The model under review builds one solid part; all positions refer to its coordinate system, in mm. Coordinates: 2 decimals unless noted, no trailing zeros. Use one line per item in the form item = value.
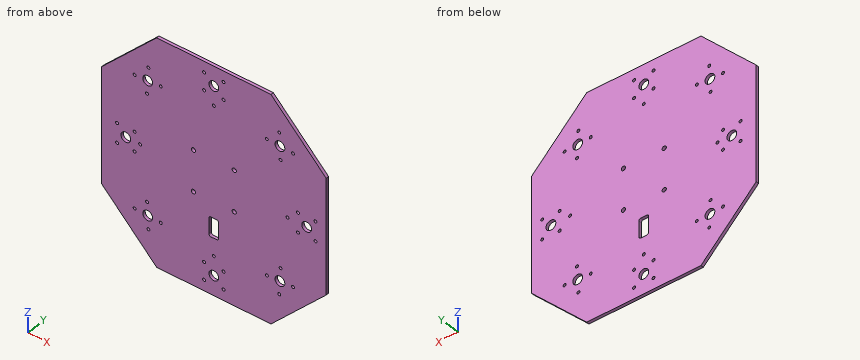
from build123d import *

# Parameters (mm, degrees)
SKETCH1_W                        = 230
SKETCH1_H                        = 230
BOSS_EXTRUDE1_DEPTH              = 3
CHAMFER2_START                   = -1
CHAMFER2_OUTLINE_W               = 82
CHAMFER2_OUTLINE_H               = 3
CHAMFER2_DEPTH                   = 40.999969952
CHAMFER3_START                   = -164
CHAMFER3_OUTLINE_W               = 83
CHAMFER3_OUTLINE_H               = 3
CHAMFER3_DEPTH                   = 41.365410279
CHAMFER4_START                   = 285.269149394
CHAMFER4_OUTLINE_W               = 82
CHAMFER4_OUTLINE_H               = 3
CHAMFER4_DEPTH                   = 40.730850606
CHAMFER5_START                   = 122.634589721
CHAMFER5_OUTLINE_W               = 83
CHAMFER5_OUTLINE_H               = 3
CHAMFER5_DEPTH                   = 41.365410279
F_11_64_0_17188_DIAMETER_HOLE1_D = 4.365752
CUT_EXTRUDE3_DEPTH               = 326.28295375
FILLET9_R                        = 2
FILLET10_R                       = 2
FILLET11_R                       = 2
FILLET12_R                       = 2
F_10_0MM_DOWEL_HOLE1_D           = 10
F_3_0MM_DOWEL_HOLE1_D            = 3
F_3_0MM_DOWEL_HOLE2_D            = 3


with BuildPart() as part:
    # Sketch1 → Boss-Extrude1 (new body)
    with BuildSketch(Plane(origin=(0, 0, 0), x_dir=(1, 0, 0), z_dir=(0, 1, 0))):
        with Locations((115, 115)):
            Rectangle(SKETCH1_W, SKETCH1_H)
    extrude(amount=BOSS_EXTRUDE1_DEPTH)

    # Chamfer2: read off the stored shape, not the designer's step
    # Chamfer2 outline → Chamfer2 (cut)
    with BuildSketch(Plane(origin=(0, 0, 0), x_dir=(0.7071067811865474, 0, 0.7071067811865477), z_dir=(0.7071067811865476, 0, -0.7071067811865476)).offset(CHAMFER2_START)):
        with Locations((0, -1.5)):
            Rectangle(CHAMFER2_OUTLINE_W, CHAMFER2_OUTLINE_H)
    extrude(amount=CHAMFER2_DEPTH, mode=Mode.SUBTRACT)

    # Chamfer3: read off the stored shape, not the designer's step
    # Chamfer3 outline → Chamfer3 (cut)
    with BuildSketch(Plane(origin=(0, 0, 0), x_dir=(0.7071067811865474, 0, -0.7071067811865477), z_dir=(0.7071067811865476, 0, 0.7071067811865476)).offset(CHAMFER3_START)):
        with Locations((162.5, 1.5)):
            Rectangle(CHAMFER3_OUTLINE_W, CHAMFER3_OUTLINE_H)
    extrude(amount=CHAMFER3_DEPTH, mode=Mode.SUBTRACT)

    # Chamfer4: read off the stored shape, not the designer's step
    # Chamfer4 outline → Chamfer4 (cut)
    with BuildSketch(Plane(origin=(0, 0, 0), x_dir=(0.7071067811865474, 0, 0.7071067811865477), z_dir=(0.7071067811865476, 0, -0.7071067811865476)).offset(CHAMFER4_START)):
        with Locations((0, -1.5)):
            Rectangle(CHAMFER4_OUTLINE_W, CHAMFER4_OUTLINE_H)
    extrude(amount=CHAMFER4_DEPTH, mode=Mode.SUBTRACT)

    # Chamfer5: read off the stored shape, not the designer's step
    # Chamfer5 outline → Chamfer5 (cut)
    with BuildSketch(Plane(origin=(0, 0, 0), x_dir=(0.7071067811865471, 0, -0.707106781186548), z_dir=(0.707106781186548, 0, 0.707106781186547)).offset(CHAMFER5_START)):
        with Locations((162.5, 1.5)):
            Rectangle(CHAMFER5_OUTLINE_W, CHAMFER5_OUTLINE_H)
    extrude(amount=CHAMFER5_DEPTH, mode=Mode.SUBTRACT)

    # 11/64 (0.17188) Diameter Hole1 (through all)
    with Locations(Plane(origin=(0, 3, 0), x_dir=(1, 0, 0), z_dir=(0, 1, 0))):
        with Locations((94.140349955, 135.859650045), (135.859650045, 135.859650045), (135.859650045, 94.140349955), (94.140349955, 94.140349955)):
            Hole(F_11_64_0_17188_DIAMETER_HOLE1_D / 2)

    # Sketch11 → Cut-Extrude3 (cut, through all)
    with BuildSketch(Plane(origin=(0, 3, 0), x_dir=(1, 0, 0), z_dir=(0, 1, 0))):
        Polygon((115, 152.5), (120, 152.5), (120, 172.5), (110, 172.5), (110, 152.5), align=None)
    extrude(amount=-CUT_EXTRUDE3_DEPTH, mode=Mode.SUBTRACT)

    # Fillet9
    fillet9_edges = [part.edges().sort_by_distance(p)[0] for p in [
        (120, 1.5, -172.5),
    ]]
    fillet(fillet9_edges, radius=FILLET9_R)

    # Fillet10
    fillet10_edges = [part.edges().sort_by_distance(p)[0] for p in [
        (110, 1.5, -172.5),
    ]]
    fillet(fillet10_edges, radius=FILLET10_R)

    # Fillet11
    fillet11_edges = [part.edges().sort_by_distance(p)[0] for p in [
        (120, 1.5, -152.5),
    ]]
    fillet(fillet11_edges, radius=FILLET11_R)

    # Fillet12
    fillet12_edges = [part.edges().sort_by_distance(p)[0] for p in [
        (110, 1.5, -152.5),
    ]]
    fillet(fillet12_edges, radius=FILLET12_R)

    # Ø10.0mm Dowel Hole1 (through all)
    with Locations(Plane(origin=(0, 3, 0), x_dir=(1, 0, 0), z_dir=(0, 1, 0))):
        with Locations((210, 115), (182.623866908, 182.623866908), (182.623866908, 47.376133092), (115, 20), (47.376133092, 47.376133092), (25, 115), (47.376133092, 182.623866908), (115, 210)):
            Hole(F_10_0MM_DOWEL_HOLE1_D / 2)

    # Ø3.0mm Dowel Hole1 (through all)
    with Locations(Plane(origin=(0, 0, 0), x_dir=(-1, 0, 0), z_dir=(0, -1, 0))):
        with Locations((-201.05, 124.95), (-201.05, 105.05), (-218.95, 124.95), (-218.95, 105.05), (-183.330973689, 60.740451256), (-169.259548744, 46.669026311), (-181.916760127, 34.011814928), (-195.988185072, 48.083239873), (-183.330973689, 169.259548744), (-169.259548744, 183.330973689), (-181.916760127, 195.988185072), (-195.988185072, 181.916760127), (-124.95, 201.05), (-124.95, 218.95), (-105.05, 218.95), (-105.05, 201.05), (-60.740451256, 183.330973689), (-34.011814928, 181.916760127), (-46.669026311, 169.259548744), (-48.083239873, 195.988185072), (-16.05, 124.95), (-33.95, 105.05), (-33.95, 124.95), (-16.05, 105.05), (-60.740451256, 46.669026311), (-48.083239873, 34.011814928), (-46.669026311, 60.740451256), (-34.011814928, 48.083239873), (-105.05, 28.95), (-105.05, 11.05), (-124.95, 28.95), (-124.95, 11.05)):
            Hole(F_3_0MM_DOWEL_HOLE1_D / 2)

    # Ø3.0mm Dowel Hole2 (through all)
    with Locations(Plane(origin=(0, 3, 0), x_dir=(1, 0, 0), z_dir=(0, 1, 0))):
        with Locations((115, 190.375), (39.625, 115), (115, 39.625), (190.375, 115)):
            Hole(F_3_0MM_DOWEL_HOLE2_D / 2)


solid = part.part
Item 1: Clearance check with flat-ended pins moving along their axes: pin 1 (2.5 mm diameter, centred on x = 94.14, z = -135.86, fed in from -Y); pin 2 (1.5 mm diameter, centred on x = 28.5, y = 2, fed in from +Z). State where each tip first meets the part, or that it passes through.
Results found:
pin_1 = through
pin_2 = -27.32
Item 2: To check wall thickness, follow L1, parallel to X at y = 1.2, z = -124.95; L2, parallel to Z at x = 136, y = 2.05; L3, parallel to Z at x = 33.5, y = 1.5. State the ranges of each line that lie inside material, in increasing order. Write a range as from..to.
Results found:
L1 = 0..14.55, 17.55..32.45, 35.45..199.55, 202.55..217.45, 220.45..230
L2 = -230..-138.04, -133.68..-96.32, -91.96..0
L3 = -206.93..-183.33, -180.51..-126.38, -123.52..-106.48, -103.62..-49.49, -46.67..-23.07
Item 3: We need section A-A (y = 1.5). State how many separate pieces and enclosed holes the cut face has, plus the area to 3 significant figures.
Results found:
separate_pieces = 1
enclosed_holes = 49
area = 45,400 mm²
